Drawing for the job (mm, zero at the part's lowest x, y, z). A direction names the side the tool comes from. Coordinates: 2 decimals unless noted, no trailing zeros. Write each loop counter-clockwise with the first axis right and the second up, starting at its lowest first coordinate (ties: lowest second). Pieces come first, ordered by that corner, then holes. Notation, with made-up numbers: (28.5, 69) -> (87.5, 69) arc R21 ccw to (87.5, 81) -> close; hole circle Ø2 at (-6.5, 35). An arc over 180 degrees is marked (long way). Answer as CSV lines item,"result".
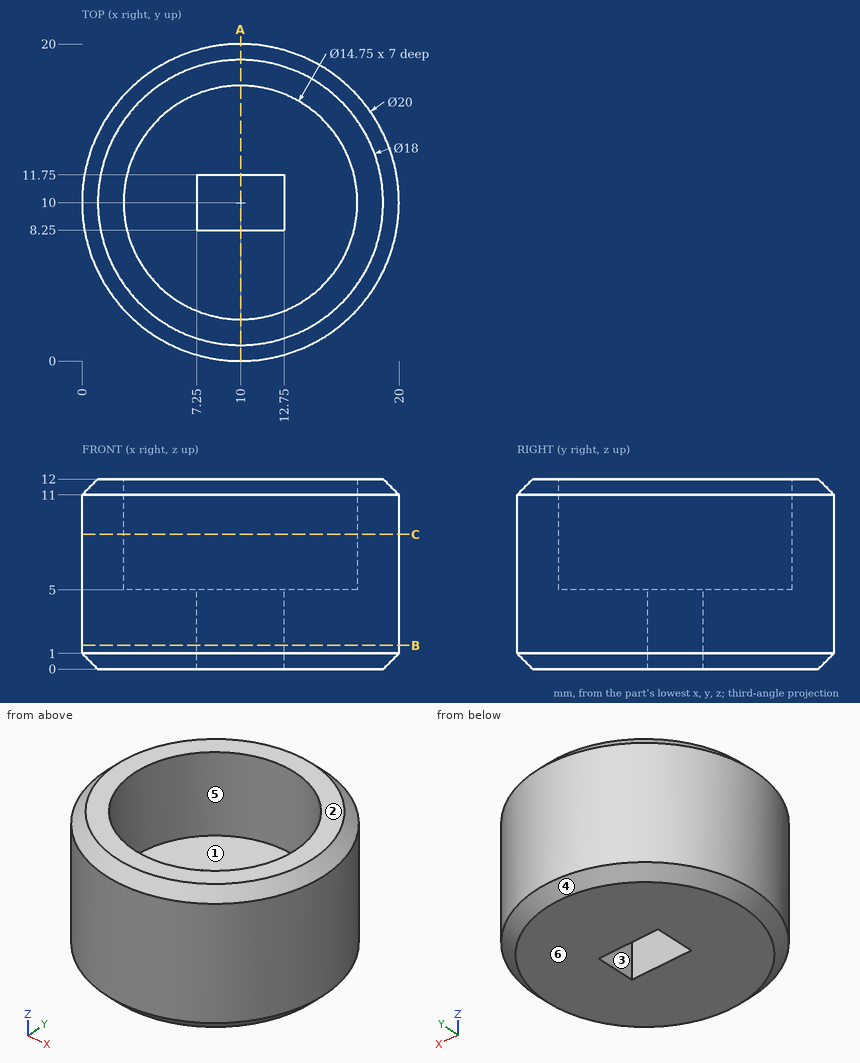
Item 1: Wall check: line 1 (Y direction, x = 10, z = 7) (3 decimals); line 2 (Z direction, x = 6.25, y = 5.25); line 3 (Y direction, x = 16.5, z = 9). Give the ranges that are in metal, low to high. Write a range as from..to.
Answer below:
line 1,"y = 0..2.625, 17.375..20"
line 2,"z = 0..5"
line 3,"y = 2.4..6.52, 13.48..17.6"
Item 2: 3-axis set-ups, long thin cutter, end or side, ignore diameter. For the marked faces 1, 2 and 3: which of +Z, -Z, +X, -X, +Y, -Y reach the whole face in a straight line?
Answer below:
face 1,"+Z"
face 2,"+Z, +X, -X, +Y, -Y"
face 3,"+Z, -Z"
Item 3: Flat gauge pins, fed straight in: pin 1 (5 mm diameter, centred on x = 13, z = 9, fed in from +Y); pin 2 (1 mm diameter, centred on y = 16, z = 7, fed in from -X); pin 3 (12 mm diameter, centred on x = 8, y = 12, fed in from +Z); pin 4 (12 mm diameter, centred on x = 10, y = 10, fed in from +Z). Where does each tip first touch, or does it go through?
Answer below:
pin 1,"stops at y = 19.99"
pin 2,"stops at x = 1.65"
pin 3,"stops at z = 12"
pin 4,"stops at z = 5"
Item 4: Saw through at B-B on z = 1.5. Give the cut face in (x, y).
Answer below:
outline,"circle Ø20 at (10, 10); hole (7.25, 8.25) -> (12.75, 8.25) -> (12.75, 11.75) -> (7.25, 11.75) -> close"
Item 5: Two-plate mould, pull along X, no slides. Class the marked faces 4, 5 and 6: pulls with the +X half, pulls with the -X half, needs draft (parallel to the pull), parting line crosses it, or undercut.
Answer below:
face 4,"parting line crosses it"
face 5,"undercut"
face 6,"needs draft"
Item 6: Saw through at C-C on z = 8.5. Give the cut face in (x, y) (3 decimals).
Answer below:
outline,"circle Ø20 at (10, 10); hole circle Ø14.75 at (10, 10)"
Item 7: Saw through at A-A on x = 10. Give the cut face in (y, z) (3 decimals), and give its area (3 significant figures).
Answer below:
outline,"(0, 1) -> (1, 0) -> (8.25, 0) -> (8.25, 5) -> (2.625, 5) -> (2.625, 12) -> (1, 12) -> (0, 11) -> close; (11.75, 0) -> (19, 0) -> (20, 1) -> (20, 11) -> (19, 12) -> (17.375, 12) -> (17.375, 5) -> (11.75, 5) -> close"
area,"117 mm2"
